Model file for the job. Use its own axes, mm. A direction names the side the tool comes from. Coordinates: 2 decimals unless noted, no trailing zeros. Write each loop counter-clockwise with the first axis right and the second up, starting at its lowest first coordinate (ties: lowest second). Pieces come first, ordered by that corner, then holes. Notation, with made-up numbers: (31, -24) -> (79, -24) arc R22 cw to (79, -13) -> close; hole circle Ø7 at (33.5, -28). An arc over 180 degrees is marked (long way). Answer as a JSON object with one key per item and string values. Group by question number.
from build123d import *

# Parameters (mm, degrees)
F1_DEPTH      = 23
F3_DEPTH      = 1.5
F6_DEPTH      = 16
F6_DEPTH_BACK = 5
F12_DEPTH     = 5


with BuildPart() as f1:
    # F0 (on Top) → F1 (new body)
    with BuildSketch(Plane.XY):
        with BuildLine():
            ThreePointArc((-2, -19), (-0.5857864376, -18.4142135624), (0, -17))
            Line((0, -17), (0, -6))
            Line((0, -6), (5.0035188667, -3.351078247))
            ThreePointArc((5.0035188667, -3.351078247), (5.3560027951, -3.039121038), (5.5267233597, -2.600467748))
            ThreePointArc((5.5267233597, -2.600467748), (6.5249806021, -0.7418373889), (8.5, 0))
            ThreePointArc((8.5, 0), (10.4750193979, -0.7418373889), (11.4732766403, -2.600467748))
            ThreePointArc((11.4732766403, -2.600467748), (11.6439972049, -3.039121038), (11.9964811333, -3.351078247))
            Line((11.9964811333, -3.351078247), (17, -6))
            Line((17, -6), (17, -17))
            ThreePointArc((17, -17), (17.5857864376, -18.4142135624), (19, -19))
            Line((19, -19), (19, -6))
            ThreePointArc((19, -6), (18.7134104706, -4.9683873987), (17.9357754408, -4.2324241673))
            Line((17.9357754408, -4.2324241673), (14.0709253105, -2.1863270395))
            ThreePointArc((14.0709253105, -2.1863270395), (13.5173932527, -1.7536531412), (13.1476433938, -1.156250862))
            ThreePointArc((13.1476433938, -1.156250862), (11.3090260154, 1.1363477665), (8.5, 2))
            ThreePointArc((8.5, 2), (5.6909739846, 1.1363477665), (3.8523566062, -1.156250862))
            ThreePointArc((3.8523566062, -1.156250862), (3.4826067473, -1.7536531412), (2.9290746895, -2.1863270395))
            Line((2.9290746895, -2.1863270395), (-0.9357754408, -4.2324241673))
            ThreePointArc((-0.9357754408, -4.2324241673), (-1.7134104706, -4.9683873987), (-2, -6))
            Line((-2, -6), (-2, -19))
        make_face()
    extrude(amount=F1_DEPTH)

    # F2 (on face) → F3 (join)
    with BuildSketch(Plane(origin=(0, 0, 0), x_dir=(1, 0, 0), z_dir=(0, 0, -1))):
        with BuildLine():
            Line((0, 10.5), (0, 6))
            Line((0, 6), (5.0035188667, 3.351078247))
            ThreePointArc((5.0035188667, 3.351078247), (5.3560027951, 3.039121038), (5.5267233597, 2.600467748))
            Line((5.5267233597, 2.600467748), (5.5267233597, 8.5))
            ThreePointArc((5.5267233597, 8.5), (4.9409369221, 9.9142135624), (3.5267233597, 10.5))
            Line((3.5267233597, 10.5), (0, 10.5))
        make_face()
        with BuildLine():
            Line((11.4732766403, 8.5), (11.4732766403, 2.600467748))
            ThreePointArc((11.4732766403, 2.600467748), (11.6439972049, 3.039121038), (11.9964811333, 3.351078247))
            Line((11.9964811333, 3.351078247), (17, 6))
            Line((17, 6), (17, 10.5))
            Line((17, 10.5), (13.4732766403, 10.5))
            ThreePointArc((13.4732766403, 10.5), (12.0590630779, 9.9142135624), (11.4732766403, 8.5))
        make_face()
    extrude(amount=-F3_DEPTH)


with BuildPart() as f6:
    # F5 (on Front) → F6 (new body, two sides)
    with BuildSketch(Plane.XZ) as f6_sk:
        with BuildLine():
            Line((-0.1767575833, 17.5), (-0.1767575833, 12.5))
            Line((-0.1767575833, 12.5), (0, 12.5))
            Line((0, 12.5), (2.7940490758, 12.5))
            add(Edge.make_bspline(
                [(2.7940490758, 12.5), (5.0035188667, 12.5), (5.0035188667, 15), (5.0035188667, 17.5), (2.7940490758, 17.5)],
                knots=[0, 0, 0, 1.5707963268, 1.5707963268, 3.1415926536, 3.1415926536, 3.1415926536], degree=2, weights=[1, 0.7071067812, 1, 0.7071067812, 1]))
            Line((2.7940490758, 17.5), (0, 17.5))
            Line((0, 17.5), (-0.1767575833, 17.5))
        make_face()
    extrude(amount=F6_DEPTH)
    extrude(f6_sk.sketch, amount=-F6_DEPTH_BACK)


with BuildPart() as f8_1:
    # F8: instance of F6
    add(f6.part.mirror(Plane.YZ.offset(8.5)))


with BuildPart() as f1_1:
    add(f1.part)

    # F9: cut F8_1, F6
    add(f8_1.part, mode=Mode.SUBTRACT)
    add(f6.part, mode=Mode.SUBTRACT)

    # F11 (on offset) → F12 (join)
    with BuildSketch(Plane.XY.offset(12.5)):
        with BuildLine():
            ThreePointArc((0, -17), (0.0635083269, -16.5), (0, -16))
            Line((0, -16), (0, -17))
        make_face()
    extrude(amount=F12_DEPTH)

    # F13: F1 across plane


with BuildPart() as f1_2:
    add(f1_1.part)
    add(f1_1.part.mirror(Plane.YZ.offset(8.5)))


solid = f1_2.part
(1) 3-axis set-ups, long thin cutter, end or side, ignore diameter. For faces 4 (the face through (16.937, -16.507, 14.965)), 5 (the face through (5, -3, 23)), 6 (the face through (17.57, -18.4, 11.34)), 7 (the face through (3, -7, 1.5)): which of +Z, -Z, +X, -X, +Y, -Y reach the whole face in a straight line?
(2) Cut at C-C on x = 15.5. List the corners of the cut face in (y, z), plus the area to 3 significant figures.
(3) Cut at D-D on y = -9.25. List the corners of the cut face in (x, z).
(4) Pin check, flat tips, straight feed: pin 1 (0.8 mm diameter, centred on x = 1.5, z = 0.5, fed in from -Y); pin 2 (1.5 mm diameter, centred on x = 2, y = -11, fed in from +Z); pin 3 (1 mm diameter, centred on y = -4.5, z = 2.5, fed in from +X). Stop position of each tip, or through.
(5) Cut at A-A on y = -13.75. List the corners of the cut face in (x, z), plus the area to 3 significant figures.
(6) Cut at B-B on z = 5.5. List the corners of the cut face in (x, y), plus the area to 3 significant figures.
(7) Wall check: probe 1 along X at (y, z) = (-16, 11.75); probe 2 along X at (y, z) = (-14.75, 15); probe 3 along Z at (x, y) = (15.5, -4). Give the ranges that are in metal, low to high.
(8) Pull direction X, two halves, no side cores. Call faces 1 (the face through (-2, -12, 11)), 2 (the face through (18.72, -4.98, 11.34)), 3 (the face through (16.6, -5.6, 12.5)): released by +X, released by -X, zero draft, split by the parting line, or undercut.
Results found:
{
 "1": {"face 4": "+Z, -Z", "face 5": "+Z, +X, -X, +Y, -Y", "face 6": "+Z, -Z, -Y", "face 7": "+Z, -Y"},
 "2": {"outline": "(-10.5, 0) -> (-2.94, 0) -> (-2.94, 12.5) -> (-5.21, 12.5) -> (-5.21, 1.5) -> (-10.5, 1.5) -> close; (-5.21, 17.5) -> (-2.94, 17.5) -> (-2.94, 23) -> (-5.21, 23) -> close", "area": "48.7 mm²"},
 "3": {"outline": "(-2, 0) -> (5.38, 0) -> (5.38, 1.5) -> (0, 1.5) -> (0, 12.5) -> (-0.18, 12.5) -> (-0.18, 17.5) -> (0, 17.5) -> (0, 23) -> (-2, 23) -> close; (11.62, 0) -> (19, 0) -> (19, 23) -> (17, 23) -> (17, 17.5) -> (17.18, 17.5) -> (17.18, 12.5) -> (17, 12.5) -> (17, 1.5) -> (11.62, 1.5) -> close"},
 "4": {"pin 1": "stops at y = -10.5", "pin 2": "stops at z = 1.5", "pin 3": "stops at x = 18.73"},
 "5": {"outline": "(-2, 0) -> (0, 0) -> (0, 12.5) -> (-0.18, 12.5) -> (-0.18, 17.5) -> (0, 17.5) -> (0, 23) -> (-2, 23) -> close; (17, 0) -> (19, 0) -> (19, 23) -> (17, 23) -> (17, 17.5) -> (17.18, 17.5) -> (17.18, 12.5) -> (17, 12.5) -> close", "area": "90.2 mm²"},
 "6": {"outline": "(-2, -19) arc R2 ccw to (0, -17) -> (0, -6) -> (5, -3.35) arc R1 ccw to (5.53, -2.6) arc R3 cw to (11.47, -2.6) arc R1 ccw to (12, -3.35) -> (17, -6) -> (17, -17) arc R2 ccw to (19, -19) -> (19, -6) arc R2 ccw to (17.94, -4.23) -> (14.07, -2.19) arc R2 cw to (13.15, -1.16) arc R5 ccw to (3.85, -1.16) arc R2 cw to (2.93, -2.19) -> (-0.94, -4.23) arc R2 ccw to (-2, -6) -> close", "area": "100 mm²"},
 "7": {"probe 1": "x = -2 to 0, 17 to 19", "probe 2": "x = -2 to -0.18, 17.18 to 19", "probe 3": "z = 0 to 12.5, 17.5 to 23"},
 "8": {"face 1": "released by -X", "face 2": "released by +X", "face 3": "undercut"}
}
